```python
from build123d import *

# Parameters (mm, degrees)
SKETCH1_W           = 75
SKETCH1_H           = 115
BOSS_EXTRUDE1_DEPTH = 5
BOSS_EXTRUDE2_DEPTH = 115
FILLET1_R           = 2
SKETCH5_W           = 75
SKETCH5_H           = 19.75
BOSS_EXTRUDE3_DEPTH = 5
FILLET2_R           = 10
FILLET3_R           = 2


with BuildPart() as part:
    # Sketch1 → Boss-Extrude1 (new body)
    with BuildSketch(Plane.XY):
        Rectangle(SKETCH1_W, SKETCH1_H)
    extrude(amount=BOSS_EXTRUDE1_DEPTH)

    # Sketch4 → Boss-Extrude2 (add)
    with BuildSketch(Plane(origin=(0, 57.5, 0), x_dir=(1, 0, 0), z_dir=(0, 1, 0))):
        Polygon((-5.75, -5), (5.75, -5), (20.5, -19.75), (-20.5, -19.75), align=None)
    extrude(amount=-BOSS_EXTRUDE2_DEPTH)

    # Fillet1
    fillet1_edges = [part.edges().sort_by_distance(p)[0] for p in [
        (5.75, 0, 5),
        (20.5, 0, 19.75),
        (-20.5, 0, 19.75),
        (-5.75, 0, 5),
    ]]
    fillet(fillet1_edges, radius=FILLET1_R)

    # Sketch5 → Boss-Extrude3 (add)
    with BuildSketch(Plane(origin=(0, 57.5, 0), x_dir=(1, 0, 0), z_dir=(0, 1, 0))):
        with Locations((0, -9.875)):
            Rectangle(SKETCH5_W, SKETCH5_H)
    extrude(amount=BOSS_EXTRUDE3_DEPTH)

    # Fillet2
    fillet2_edges = [part.edges().sort_by_distance(p)[0] for p in [
        (-37.5, 60, 19.75),
        (37.5, 60, 19.75),
        (37.5, -57.5, 2.5),
        (-37.5, -57.5, 2.5),
    ]]
    fillet(fillet2_edges, radius=FILLET2_R)

    # Fillet3
    fillet3_edges = [part.edges().sort_by_distance(p)[0] for p in [
        (-37.5, 5, 5),
        (-13.125, -57.5, 12.375),
        (13.125, -57.5, 12.375),
        (19.039213562, -57.5, 5),
        (0, -57.5, 19.75),
        (-17.51933194, -57.5, 18.515366865),
        (17.51933194, -57.5, 18.515366865),
        (-8.73066806, -57.5, 6.234633135),
        (8.73066806, -57.5, 6.234633135),
        (-37.5, 57.5, 7.375),
        (21.585786438, 57.5, 19.75),
        (-37.5, 62.5, 4.875),
        (0, 62.5, 19.75),
        (-21.585786438, 57.5, 19.75),
        (-34.571067812, 57.5, 16.821067812),
        (37.5, 62.5, 4.875),
        (34.571067812, 62.5, 16.821067812),
        (-34.571067812, 62.5, 16.821067812),
        (37.5, 57.5, 7.375),
        (37.5, 5, 5),
        (34.571067812, 57.5, 16.821067812),
        (-19.039213562, -57.5, 5),
        (34.571067812, -54.571067812, 5),
        (-34.571067812, -54.571067812, 5),
    ]]
    fillet(fillet3_edges, radius=FILLET3_R)


solid = part.part
```
Here's how the part is built. I have some questions about the finished solid (model axes, mm). A direction names the side the tool comes from. Give positions to 0.01 mm unless a question says otherwise; leave off trailing zeros. Order: outer loops, then holes, each group sorted by start corner. A loop starts at its lowest first (then second) coordinate and runs counter-clockwise, first axis right, second up. Notation, with made-up numbers: M 27.5,79 L 38.5,79 A32 cw 38.5,117 Z; hole C 20,-7 d4. An arc over 180 degrees is marked long. Use a Markdown table: item, result. Add a question column.
1. I need wall thicknesses on probe 1 along Z at (x, y) = (-31, -17.5); probe 2 along X at (y, z) = (-13, 18); probe 3 along Y at (x, z) = (-24, 9.5). Which ranges of each line are inside material? Lowest first, please. Write a range as from..to.
2. If we mould it in two halves opening along Z, with no side actions, what happens to faces 4 (the cylindrical face through (-34.65, 60.01, 16.74)), 5 (the flat face through (37.5, 6, 2)), 6 (the cylindrical face through (8.744, 0.209, 6.204)), 7 (the cylindrical face through (17.532, 1.195, 18.485))? For each: +Z half, -Z half, draft (parallel to the pull), parting line (faces both ways), or undercut.
3. Suppose I cut it at A-A (y = -8). List the corners of the cut face in (x, z) for me, and give its area (3 significant figures).
4. Suppose I cut it at B-B (x = -25). List the corners of the cut face in (y, z) for me.
5. On a 3-axis mill with a long thin cutter (end or side, diameter ignored), from which of +Z, -Z, +X, -X, +Y, -Y can I reach the whole of each face in a straight line? I mean faces 1 (the cylindrical face through (-12.64, -56.93, 12.74)), 2 (the flat face through (13.07, 1.79, 12.32)), 3 (the flat face through (-1, 2, 0)). Say none if no direction works.
6. For pin 1 Ø1 at (x, y) = (-26, -8) entering from +Z; pin 2 Ø5 at (y, z) = (0, 6) entering from +X; pin 3 Ø4 at (x, z) = (-28.5, 8.5) entering from -Y, each with a flat end and sliding along its axis, tell me the tip position at first contact or that it passes through.
Results list:
| question | item | result |
|---|---|---|
| 1 | probe 1 | z = 0..5 |
| 1 | probe 2 | x = -17.66..17.66 |
| 1 | probe 3 | y = 57.5..62.5 |
| 2 | face 4 | +Z half |
| 2 | face 5 | draft |
| 2 | face 6 | undercut |
| 2 | face 7 | undercut |
| 3 | outline | M -37.5,0 L 37.5,0 L 37.5,3 A2 ccw 35.5,5 L 10.58,5 A2 cw 9.16,8.41 L 17.09,16.34 A2 ccw 15.67,19.75 L -15.67,19.75 A2 ccw -17.09,16.34 L -9.16,8.41 A2 cw -10.58,5 L -35.5,5 A2 ccw -37.5,3 Z |
| 3 | area | 760 mm² |
| 4 | outline | M -57.5,0 L 62.5,0 L 62.5,17.75 A2 ccw 60.5,19.75 L 59.5,19.75 A2 ccw 57.5,17.75 L 57.5,5 L -55.5,5 A2 ccw -57.5,3 Z |
| 5 | face 1 | -X, -Y |
| 5 | face 2 | +X, -Y |
| 5 | face 3 | -Z, +X, -X, +Y, -Y |
| 6 | pin 1 | stops at z = 5 |
| 6 | pin 2 | stops at x = 37.44 |
| 6 | pin 3 | stops at y = 57.5 |
